Can you work these out from the model? Positions are in its coordinate system, mm. Face numbers are marked on the shaded views. Coordinates: 2 decimals unless noted, no trailing zeros. Loops run counter-clockwise (first coordinate to the right, second up) from the corner with the lowest first, then second, coordinate; pieces in that order, holes last.
```python
from build123d import *

# Parameters (mm, degrees)
SKETCH2_R           = 20
SKETCH2_R_2         = 18
BOSS_EXTRUDE1_DEPTH = 200
SKETCH2_3_R         = 21
SKETCH2_3_R_2       = 20
BOSS_EXTRUDE2_DEPTH = 4
BOSS_EXTRUDE3_START = 54
SKETCH2_4_R         = 21
SKETCH2_4_R_2       = 20
BOSS_EXTRUDE3_DEPTH = 4


with BuildPart() as part:
    # Sketch2 → Boss-Extrude1 (new body)
    with BuildSketch(Plane.XY):
        Circle(SKETCH2_R)
        Circle(SKETCH2_R_2, mode=Mode.SUBTRACT)
    extrude(amount=BOSS_EXTRUDE1_DEPTH)

    # Sketch2<3> → Boss-Extrude2 (add)
    with BuildSketch(Plane.XY):
        Circle(SKETCH2_3_R)
        Circle(SKETCH2_3_R_2, mode=Mode.SUBTRACT)
    extrude(amount=BOSS_EXTRUDE2_DEPTH)

    # Sketch2<4> → Boss-Extrude3 (add)
    with BuildSketch(Plane.XY.offset(BOSS_EXTRUDE3_START)):
        Circle(SKETCH2_4_R)
        Circle(SKETCH2_4_R_2, mode=Mode.SUBTRACT)
    extrude(amount=BOSS_EXTRUDE3_DEPTH)


solid = part.part
```
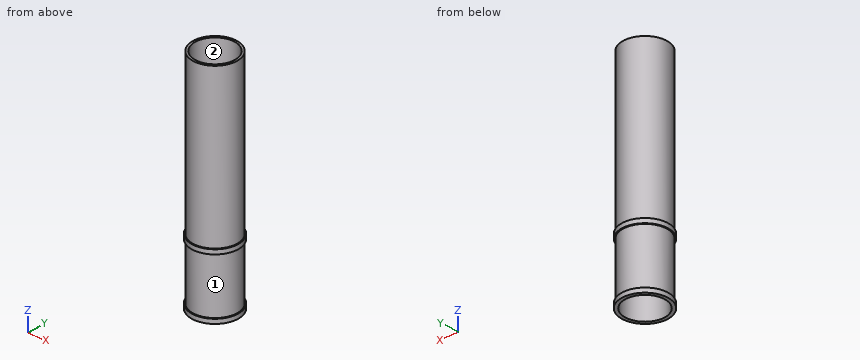
Item 1: I need wall thicknesses on line 1 along Y through (x, z) = (0, 74); line 2 along Z through (x, y) = (9.5, -18.5); line 3 along X through (y, z) = (15, 135). Which ranges of each line are inside material? Lowest first, please.
Results are:
line 1: y = -20 to -18, 18 to 20
line 2: z = 0 to 4, 54 to 58
line 3: x = -13.23 to -9.95, 9.95 to 13.23
Item 2: I'm going to push flat-ended pins straight in: P1, Ø2, axis at x = 10, z = 151, coming from the +Y side; P2, Ø5, axis at y = -2.5, z = 143.5, coming from the -X side; P3, Ø4, axis at x = 13.5, z = 140, coming from the +Y side. Where does each tip first touch, or does it pass through?
Results are:
P1: stops at y = 17.86
P2: stops at x = -20
P3: stops at y = 16.36
Item 3: Suppose I cut it at C-C, the plane z = 87.5. Please give me the cut outline in (x, y).
Results are:
outline: circle Ø40 at (0, 0); hole circle Ø36 at (0, 0)
Item 4: We'd pull the mould along Y, two halves only. Please class the marked faces 1 and 2: +Y half, -Y half, draft (parallel to the pull), parting line (faces both ways), or undercut.
Results are:
face 1: parting line
face 2: undercut
Item 5: Suppose I cut it at A-A, the plane x = 0. Please give me the cut outline in (y, z).
Results are:
outline: (-21, 0) - (-18, 0) - (-18, 200) - (-20, 200) - (-20, 58) - (-21, 58) - (-21, 54) - (-20, 54) - (-20, 4) - (-21, 4) - close; (18, 0) - (21, 0) - (21, 4) - (20, 4) - (20, 54) - (21, 54) - (21, 58) - (20, 58) - (20, 200) - (18, 200) - close
